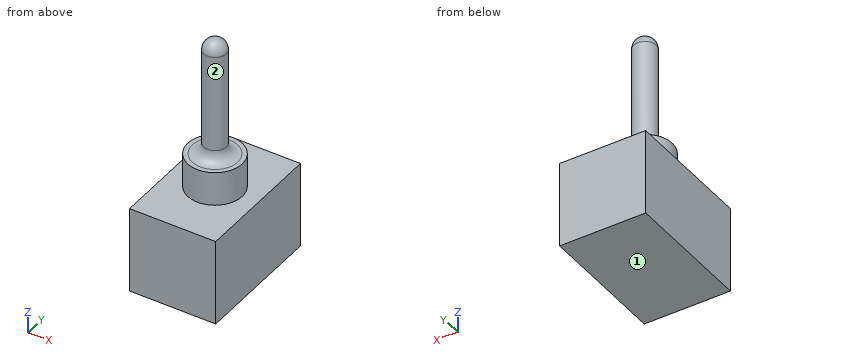
```python
from build123d import *

# Parameters (mm, degrees)
ESQUISSE1_W        = 19
ESQUISSE1_H        = 29
BOSS_EXTRU_1_DEPTH = 19
ESQUISSE3_R        = 6
BOSS_EXTRU_2_DEPTH = 7.5
ESQUISSE4_R        = 2.5
BOSS_EXTRU_3_DEPTH = 26.5
CONG_3_R           = 2.5


with BuildPart() as part:
    # Esquisse1 → Boss.-Extru.1 (new body)
    with BuildSketch(Plane.XY):
        with Locations((-54.306805708, 14.681818182)):
            Rectangle(ESQUISSE1_W, ESQUISSE1_H)
    extrude(amount=BOSS_EXTRU_1_DEPTH)

    # Esquisse3 → Boss.-Extru.2 (add)
    with BuildSketch(Plane.XY.offset(19)):
        with Locations((-54.306805708, 14.681818182)):
            Circle(ESQUISSE3_R)
    extrude(amount=BOSS_EXTRU_2_DEPTH)

    # Esquisse4 → Boss.-Extru.3 (add)
    with BuildSketch(Plane.XY.offset(26.5)):
        with Locations((-54.306805708, 14.681818182)):
            Circle(ESQUISSE4_R)
    extrude(amount=BOSS_EXTRU_3_DEPTH)

    # Congé3
    cong_3_edges = [part.edges().sort_by_distance(p)[0] for p in [
        (-56.806805708, 14.681818182, 26.5),
        (-56.806805708, 14.681818182, 53),
    ]]
    fillet(cong_3_edges, radius=CONG_3_R)


solid = part.part
```
The listing builds one solid part. Answer for the finished solid, in the listing's coordinates (mm). Face numbers are marked on the shaded views. A direction names the side the tool comes from. Round coordinates to 2 decimals unless told otherwise and drop trailing zeros. Loops run counter-clockwise (first coordinate to the right, second up) from the corner with the lowest first, then second, coordinate; pieces in that order, holes last.
Q1. Section A-A, the plane y = 7.5 is taken. Determine the outline of the cut face in (x, z).
Q2. Find the intervals of material crossed by line 1 (X direction, y = 14.5, z = 37); line 2 (Z direction, x = -59.75, y = 20.5); line 3 (Z direction, x = -59.5, y = 15.25), in increasing order.
Q3. Section C-C, the plane z = 32.5 is taken. Determine the outline of the cut face in (x, y).
Q4. Given pin 1 Ø1 at (x, y) = (-51, 22.5) entering from +Z; pin 2 Ø10 at (x, y) = (-59.5, 6) entering from +Z, each flat-ended and moving along its own axis, determine where each tip first touches the part or whether it passes through.
Q5. Which of the six approach directions +Z, -Z, +X, -X, +Y, -Y give full straight-line access (tool end or side, diameter ignored) to the marked faces 1 and 2?
Q6. Section D-D, the plane z = 22.5 is taken. Determine the outline of the cut face in (x, y).
Q7. Section B-B, the plane x = -47.75 is taken. Determine the outline of the cut face in (y, z).
Completed:
1. outline: (-63.81, 0) - (-44.81, 0) - (-44.81, 19) - (-63.81, 19) - close
2. line 1: x = -56.8 to -51.81
2. line 2: z = 0 to 19
2. line 3: z = 0 to 26.5
3. outline: circle Ø5 at (-54.31, 14.68)
4. pin 1: stops at z = 19
4. pin 2: stops at z = 26.5
5. face 1: -Z, +X, -X, +Y, -Y
5. face 2: +Z
6. outline: circle Ø12 at (-54.31, 14.68)
7. outline: (0.18, 0) - (29.18, 0) - (29.18, 19) - (0.18, 19) - close
